```python
from build123d import *

# Parameters (mm, degrees)
SKETCH1_R           = 66.675
BOSS_EXTRUDE1_DEPTH = 3.175
CUT_EXTRUDE4_DEPTH  = 3.175
SKETCH10_R          = 2.0955
CUT_EXTRUDE7_DEPTH  = 4.175


with BuildPart() as part:
    # Sketch1 → Boss-Extrude1 (new body)
    with BuildSketch(Plane(origin=(0, 0, 0), x_dir=(1, 0, 0), z_dir=(0, 1, 0))):
        with BuildLine():
            Line((-110.396900432, 76.2), (-298.45, 76.2))
            ThreePointArc((-298.45, 76.2), (-334.371024484, 61.321024484), (-349.25, 25.4))
            Line((-349.25, 25.4), (-349.25, -25.4))
            ThreePointArc((-349.25, -25.4), (-334.371024484, -61.321024484), (-298.45, -76.2))
            Line((-298.45, -76.2), (-110.396900432, -76.2))
            ThreePointArc((-110.396900432, -76.2), (-92.606633854, -79.41695244), (-77.069534264, -88.660377358))
            ThreePointArc((-77.069534264, -88.660377358), (0, -117.475), (77.069534264, -88.660377358))
            ThreePointArc((77.069534264, -88.660377358), (92.606633854, -79.41695244), (110.396900432, -76.2))
            Line((110.396900432, -76.2), (298.45, -76.2))
            ThreePointArc((298.45, -76.2), (334.371024484, -61.321024484), (349.25, -25.4))
            Line((349.25, -25.4), (349.25, 25.4))
            ThreePointArc((349.25, 25.4), (334.371024484, 61.321024484), (298.45, 76.2))
            Line((298.45, 76.2), (110.396900432, 76.2))
            ThreePointArc((110.396900432, 76.2), (92.606633854, 79.41695244), (77.069534264, 88.660377358))
            ThreePointArc((77.069534264, 88.660377358), (0, 117.475), (-77.069534264, 88.660377358))
            ThreePointArc((-77.069534264, 88.660377358), (-92.606633854, 79.41695244), (-110.396900432, 76.2))
        make_face()
        Circle(SKETCH1_R, mode=Mode.SUBTRACT)
    extrude(amount=BOSS_EXTRUDE1_DEPTH)

    # Sketch7 → Cut-Extrude4 (cut)
    with BuildSketch(Plane(origin=(0, 3.175, 0), x_dir=(1, 0, 0), z_dir=(0, 1, 0))):
        with BuildLine():
            Line((-25.4, -87.56211469), (25.4, -87.56211469))
            ThreePointArc((25.4, -87.56211469), (33.3375, -95.49961469), (25.4, -103.43711469))
            Line((25.4, -103.43711469), (-25.4, -103.43711469))
            ThreePointArc((-25.4, -103.43711469), (-33.3375, -95.49961469), (-25.4, -87.56211469))
        make_face()
    extrude(amount=-CUT_EXTRUDE4_DEPTH, mode=Mode.SUBTRACT)

    # Sketch10 → Cut-Extrude7 (cut, through all)
    with BuildSketch(Plane(origin=(0, 3.175, 0), x_dir=(1, 0, 0), z_dir=(0, 1, 0))):
        with Locations((-93.6244, -26.9875)):
            Circle(SKETCH10_R)
        with Locations((-106.3244, -14.2875)):
            Circle(SKETCH10_R)
        with Locations((-93.6244, -1.5875)):
            Circle(SKETCH10_R)
        with Locations((-106.3244, 11.1125)):
            Circle(SKETCH10_R)
        with Locations((-93.6244, 23.8125)):
            Circle(SKETCH10_R)
        with Locations((93.6244, -26.9875)):
            Circle(SKETCH10_R)
        with Locations((106.3244, -14.2875)):
            Circle(SKETCH10_R)
        with Locations((93.6244, -1.5875)):
            Circle(SKETCH10_R)
        with Locations((106.3244, 11.1125)):
            Circle(SKETCH10_R)
        with Locations((93.6244, 23.8125)):
            Circle(SKETCH10_R)
    extrude(amount=-CUT_EXTRUDE7_DEPTH, mode=Mode.SUBTRACT)


solid = part.part
```
Check sheet for the modelled part. Datum: model origin and axes. Units: mm. Coordinates: 2 decimals unless noted, no trailing zeros. Loops run counter-clockwise (first coordinate to the right, second up) from the corner with the lowest first, then second, coordinate; pieces in that order, holes last.
1) Sectioned sample at C-C (y = 2.3). Count the separate pieces of the cut face and the enclosed holes in it, and give its area (3 significant figures).
2) Release check for a two-part mould opening along Z. For faces 1 (the face through (1.18, 1.57, -117.47)), 2 (the face through (63.596, 1.565, -20.027)), 3 (the face through (-334.764, 1.565, 60.924)) record: released by +Z, released by -Z, zero draft, split by the parting line, or undercut.
3) Material ranges on probe 1 along X at (y, z) = (0.2, -22); probe 2 along X at (y, z) = (0.2, 16); probe 3 along Z at (x, y) = (32.5, 1), recorded low to high.
4) Sectioned sample at A-A (x = 0). Record the boundary of the cut face in (y, z) (3 decimals), and give its area (3 significant figures).
5) Sectioned sample at D-D (x = 211). Record the boundary of the cut face in (y, z) (3 decimals).
6) Sectioned sample at B-B (z = 58). Record the boundary of the cut face in (x, y) (3 decimals).
7) Gauge pin test, flat ends, axial feed: pin 1 (5 mm diameter, centred on x = 106.32, z = -11.11, fed in from -Y); pin 2 (4 mm diameter, centred on x = -106.32, z = -11.11, fed in from -Y); pin 3 (1 mm diameter, centred on x = 189.5, y = 2, fed in from +Z); pin 4 (1 mm diameter, centred on y = 2, z = 85, fed in from -X). Record the tip position at first contact, or that the pin passes through.
Check sheet entries:
1. separate pieces: 1
1. enclosed holes: 12
1. area: 99,600 mm2
2. face 1: released by -Z
2. face 2: undercut
2. face 3: released by +Z
3. probe 1: x = -349.25 to -94.68, -92.57 to -62.94, 62.94 to 92.57, 94.68 to 349.25
3. probe 2: x = -349.25 to -107.53, -105.12 to -64.73, 64.73 to 105.12, 107.53 to 349.25
3. probe 3: z = -112.89 to -58.22, 58.22 to 91.95, 99.05 to 112.89
4. outline: (0, -117.475) - (3.175, -117.475) - (3.175, -66.675) - (0, -66.675) - close; (0, 66.675) - (3.175, 66.675) - (3.175, 87.562) - (0, 87.562) - close; (0, 103.437) - (3.175, 103.437) - (3.175, 117.475) - (0, 117.475) - close
4. area: 272 mm2
5. outline: (0, -76.2) - (3.175, -76.2) - (3.175, 76.2) - (0, 76.2) - close
6. outline: (-337.41, 0) - (-32.887, 0) - (-32.887, 3.175) - (-337.41, 3.175) - close; (32.887, 0) - (337.41, 0) - (337.41, 3.175) - (32.887, 3.175) - close
7. pin 1: stops at y = 0
7. pin 2: passes through
7. pin 3: stops at z = 76.2
7. pin 4: stops at x = -82.57
